Here's how the part is built. I have some questions about the finished solid (model axes, mm). Face numbers are marked on the shaded views. Round coordinates to 2 decimals unless told otherwise and drop trailing zeros. Write each loop counter-clockwise with the first axis right and the second up, starting at its lowest first coordinate (ties: lowest second). Pieces come first, ordered by that corner, then holes. Notation, with made-up numbers: (76.25, 25.25) - (95.25, 25.25) arc R24 cw to (95.25, 47.25) - close; hole circle Ø5 at (63, 67.5). An arc over 180 degrees is marked (long way). Write item = value, one per line. Start each with the question number.
Item 1: If we section it at B-B (y = 0): Please give me the cut outline in (x, z).
Item 2: If we section it at C-C (y = -43.5): Please give me the cut outline in (x, z) (1 decimal).
Item 3: If I drill on line 1 along Y through (x, z) = (0, 96); line 2 along Y through (x, z) = (0, 96.8); line 3 along Z through (x, y) = (2, 14.5), over which ranges is the centre line in solid material (lowest first)? Write a range as [from, to].
Item 4: For P1, Ø4, axis at x = -10.5, y = 9.5, coming from the -Z side, with a flat end and sliding along its axis, tell me the tip position at first contact or that it passes through.
Item 5: If we section it at A-A (x = 9): Please give me the cut outline in (y, z), and give its area (3 significant figures).
Item 6: Thinking about a two-plate mould opening in X: for the marked faces 1, 2 and 3, which applies, pulls with the +X half, pulls with the -X half, needs draft (parallel to the pull), parting line crosses it, or undercut?
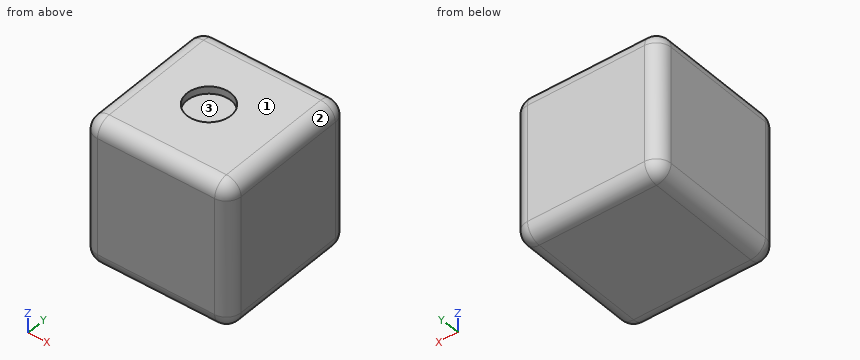
```python
from build123d import *

# Parameters (mm, degrees)
F0_W     = 100
F0_H     = 100
F1_DEPTH = 100
F2_R     = 10
F3_R     = 15
F4_DEPTH = 5


with BuildPart() as f1:
    # F0 (on Top) → F1 (new body)
    with BuildSketch(Plane.XY):
        with Locations((4.118751, 0)):
            Rectangle(F0_W, F0_H)
    extrude(amount=F1_DEPTH)

    # F2
    f2_edges = [f1.edges().sort_by_distance(p)[0] for p in [
        (4.118751, 50, 100),
        (-45.881249, 0, 100),
        (4.118751, -50, 100),
        (54.118751, 0, 100),
        (-45.881249, -50, 50),
        (54.118751, -50, 50),
        (4.118751, -50, 0),
        (54.118751, 50, 50),
        (54.118751, 0, 0),
        (-45.881249, 50, 50),
        (4.118751, 50, 0),
        (-45.881249, 0, 0),
    ]]
    fillet(f2_edges, radius=F2_R)

    # F3 (on face) → F4 (cut)
    with BuildSketch(Plane.XY.offset(100)):
        Circle(F3_R)
    extrude(amount=-F4_DEPTH, mode=Mode.SUBTRACT)


solid = f1.part
```
Reply:
q1.outline = (-45.88, 10) arc R10 ccw to (-35.88, 0) - (44.12, 0) arc R10 ccw to (54.12, 10) - (54.12, 90) arc R10 ccw to (44.12, 100) - (15, 100) - (15, 95) - (-15, 95) - (-15, 100) - (-35.88, 100) arc R10 ccw to (-45.88, 90) - close
q2.outline = (-45.2, 10) arc R9.4 ccw to (-35.9, 0.6) - (44.1, 0.6) arc R9.4 ccw to (53.5, 10) - (53.5, 90) arc R9.4 ccw to (44.1, 99.4) - (-35.9, 99.4) arc R9.4 ccw to (-45.2, 90) - close
q3.line_1 = [-48, -15], [15, 48]
q3.line_2 = [-47.33, -15], [15, 47.33]
q3.line_3 = [0, 95]
q4.P1 = 0
q5.outline = (-50, 10) arc R10 ccw to (-40, 0) - (40, 0) arc R10 ccw to (50, 10) - (50, 90) arc R10 ccw to (40, 100) - (12, 100) - (12, 95) - (-12, 95) - (-12, 100) - (-40, 100) arc R10 ccw to (-50, 90) - close
q5.area = 9,790 mm2
q6.face_1 = needs draft
q6.face_2 = pulls with the +X half
q6.face_3 = undercut
